```python
from build123d import *

# Parameters (mm, degrees)
PAD_DEPTH = 8


with BuildPart() as part:
    # Sketch → Pad (new body)
    with BuildSketch(Plane.XY):
        with BuildLine():
            Line((51.5303, 115.351058), (57.5303, 115.351058))
            Line((57.5303, 115.351058), (57.5303, 17.037153))
            ThreePointArc((-15.362291, 58), (-29.394284, -52.306558), (57.5303, 17.037153))
            Line((43.5303, 67.351058), (-15.362291, 58))
            Line((51.5303, 67.351058), (43.5303, 67.351058))
            Line((51.5303, 75.351058), (51.5303, 67.351058))
            Line((43.5303, 75.351058), (51.5303, 75.351058))
            Line((43.5303, 83.351058), (43.5303, 75.351058))
            Line((51.5303, 83.351058), (43.5303, 83.351058))
            Line((51.5303, 91.351058), (51.5303, 83.351058))
            Line((43.5303, 91.351058), (51.5303, 91.351058))
            Line((43.5303, 99.351058), (43.5303, 91.351058))
            Line((51.5303, 99.351058), (43.5303, 99.351058))
            Line((51.5303, 107.351058), (51.5303, 99.351058))
            Line((43.5303, 107.351058), (51.5303, 107.351058))
            Line((43.5303, 115.351058), (43.5303, 107.351058))
            Line((51.5303, 115.351058), (43.5303, 115.351058))
        make_face()
    extrude(amount=PAD_DEPTH)


solid = part.part
```
Source: CAD feature listing. Evaluate the final solid. Frame: model axes, mm. A direction names the side the tool comes from. Give positions to 0.01 mm unless a question says otherwise; leave off trailing zeros. Write each loop counter-clockwise with the first axis right and the second up, starting at its lowest first coordinate (ties: lowest second). Pieces come first, ordered by that corner, then holes. Notation, with made-up numbers: (74.5, -19) - (84.5, -19) arc R12 ccw to (84.5, 2) - close; hole circle Ø3 at (59.25, 53). An arc over 180 degrees is marked (long way). One line per item, written item: value. Start each with the question number.
Q1. First-contact query: pin 1 Ø4 at (x, z) = (14.5, 2.5) entering from -Y; pin 2 Ø10 at (x, y) = (-46.5, -35.5) entering from -Z; pin 3 Ø4 at (x, z) = (48, 4.5) entering from -Y; pin 4 Ø3 at (y, z) = (92.5, 4.5) entering from +X. Flat tips, straight axial feed; report the tip coordinate or a pass-through.
Q2. Draft query along Y for faces 1 (the face through (43.53, 95, 4)), 2 (the face through (47, 107.351, 4)), 3 (the face through (51, 115.351, 4)). Return one class per face: +Y half, -Y half, draft (parallel to the pull), parting line (faces both ways), or undercut.
Q3. Section query B-B, the plane y = 78.5. Return the cut outline in (x, z), then the cut area to 3 significant figures.
Q4. Section query A-A, the plane z = 5.25. Return the cut outline in (x, y).
Q5. Section query C-C, the plane x = -20. Return the cut outline in (y, z).
Q6. Material intervals for probe 1 along X at (y, z) = (87, 3.5); probe 2 along X at (y, z) = (95, 1.75); probe 3 along Y at (x, z) = (37.5, 1.75), sorted ascending. Write a range as from..to.
Q7. Set-up query: faces 4 (the face through (51.53, 87, 4)), 5 (the face through (57.53, 67, 4)), 6 (the face through (1, 9, 0)), 7 (the face through (43.53, 111, 4)). Return all of +Z, -Z, +X, -X, +Y, -Y with unobstructed straight access to the full face (end or side cutting, diameter ignored); none if empty.
Answer:
1. pin 1: stops at y = -58.68
1. pin 2: stops at z = 0
1. pin 3: stops at y = -38.52
1. pin 4: stops at x = 57.53
2. face 1: draft
2. face 2: undercut
2. face 3: +Y half
3. outline: (43.53, 0) - (57.53, 0) - (57.53, 8) - (43.53, 8) - close
3. area: 112 mm2
4. outline: (-15.36, 58) arc R60 ccw (long way) to (57.53, 17.04) - (57.53, 115.35) - (43.53, 115.35) - (43.53, 107.35) - (51.53, 107.35) - (51.53, 99.35) - (43.53, 99.35) - (43.53, 91.35) - (51.53, 91.35) - (51.53, 83.35) - (43.53, 83.35) - (43.53, 75.35) - (51.53, 75.35) - (51.53, 67.35) - (43.53, 67.35) - close
5. outline: (-56.57, 0) - (56.57, 0) - (56.57, 8) - (-56.57, 8) - close
6. probe 1: x = 51.53..57.53
6. probe 2: x = 43.53..57.53
6. probe 3: y = -46.84..66.39
7. face 4: +Z, -Z, -X
7. face 5: +Z, -Z, +X, +Y
7. face 6: -Z, +X, -X, +Y, -Y
7. face 7: +Z, -Z, -X, +Y
